Can you work these out from the model? Positions are in its coordinate system, mm. Face numbers are marked on the shaded views. A direction names the side the tool comes from. Round coordinates to 2 decimals unless told otherwise and drop trailing zeros. Write each loop counter-clockwise with the first axis right and the second up, starting at its lowest first coordinate (ties: lowest second). Pieces come first, ordered by that corner, then holes. Notation, with made-up numbers: M 0,25.5 L 47,25.5 A28 cw 47,60.5 Z; hole C 40.5,25.5 d2. An arc over 180 degrees is marked long. Answer as a JSON object with one key per item and string values. Group by question number.
1) Suppose I cut it at C-C, the plane z = 7. Write out the boundary of the cut face in (x, y), and give its area (3 significant figures).
2) I'm going to push flat-ended pins straight in: pin 1 Ø1 at (x, y) = (-10.5, -10) entering from +Z; pin 2 Ø2 at (y, z) = (18.5, 4) entering from -X; pin 3 Ø8 at (y, z) = (-21, 5) entering from -X; pin 4 Ø1.5 at (x, y) = (24, -21.5) entering from -Z. Where does each tip first touch, or does it pass through?
3) On a 3-axis mill with a long thin cutter (end or side, diameter ignored), from which of +Z, -Z, +X, -X, +Y, -Y can I reach the whole of each face in a straight line? I mean the marked faces 4, 5 and 6. Say none if no direction works.
4) Please list where these lines run through material, in increasing order: L1, parallel to Z at x = 15.5, y = 23; L2, parallel to Z at x = -6.5, y = -14.5; L3, parallel to Y at x = -7.5, z = -7.25. Write a range as [from, to].
5) Suppose I cut it at B-B, the plane x = 0. Write out the boundary of the cut face in (y, z).
6) Suppose I cut it at A-A, the plane y = 0. Write out the boundary of the cut face in (x, z), and give its area (3 significant figures).
7) If we mould it in two halves opening along X, with no side actions, what happens to the marked faces 1, 2 and 3? For each: +X half, -X half, draft (parallel to the pull), parting line (faces both ways), or undercut.
8) Suppose I cut it at D-D, the plane y = 20. Write out the boundary of the cut face in (x, z).
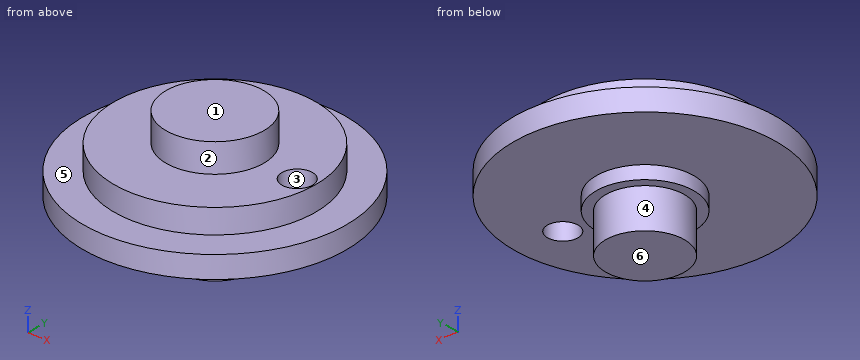
from build123d import *

# Parameters (mm, degrees)
F0_R          = 30
F1_DEPTH      = 5
F2_R          = 11.15
F3_DEPTH      = 12
F3_DEPTH_BACK = 8
F4_R          = 9
F5_DEPTH      = 9
F6_R          = 23
F7_DEPTH      = 5.5
F8_R          = 3.5
F9_DEPTH      = 12.5


with BuildPart() as f1:
    # F0 (on Top) → F1 (new body)
    with BuildSketch(Plane.XY):
        Circle(F0_R)
    extrude(amount=F1_DEPTH)

    # F2 (on face) → F3 (join, two sides)
    with BuildSketch(Plane.XY.offset(5)) as f3_sk:
        Circle(F2_R)
    extrude(amount=F3_DEPTH)
    extrude(f3_sk.sketch, amount=-F3_DEPTH_BACK)

    # F4 (on face) → F5 (join)
    with BuildSketch(Plane(origin=(0, 0, -3), x_dir=(1, 0, 0), z_dir=(0, 0, -1))):
        Circle(F4_R)
    extrude(amount=F5_DEPTH)

    # F6 (on face) → F7 (join)
    with BuildSketch(Plane.XY.offset(5)):
        Circle(F6_R)
    extrude(amount=F7_DEPTH)

    # F8 (on face) → F9 (cut, symmetric)
    with BuildSketch(Plane.XY.offset(5)):
        with Locations((19.200256, 0)):
            Circle(F8_R)
    extrude(amount=F9_DEPTH, both=True, mode=Mode.SUBTRACT)


solid = f1.part
Results:
{
 "1": {"outline": "C 0,0 d46; hole C 19.2,0 d7", "area": "1,620 mm^2"},
 "2": {"pin 1": "z = 10.5", "pin 2": "x = -24.37", "pin 3": "x = -24.72", "pin 4": "through"},
 "3": {"face 4": "-Z", "face 5": "+Z", "face 6": "-Z, +X, -X, +Y, -Y"},
 "4": {"L1": "[0, 5]", "L2": "[0, 10.5]", "L3": "[-4.97, 4.97]"},
 "5": {"outline": "M -30,0 L -11.15,0 L -11.15,-3 L -9,-3 L -9,-12 L 9,-12 L 9,-3 L 11.15,-3 L 11.15,0 L 30,0 L 30,5 L 23,5 L 23,10.5 L 11.15,10.5 L 11.15,17 L -11.15,17 L -11.15,10.5 L -23,10.5 L -23,5 L -30,5 Z"},
 "6": {"outline": "M -30,0 L -11.15,0 L -11.15,-3 L -9,-3 L -9,-12 L 9,-12 L 9,-3 L 11.15,-3 L 11.15,0 L 15.7,0 L 15.7,10.5 L 11.15,10.5 L 11.15,17 L -11.15,17 L -11.15,10.5 L -23,10.5 L -23,5 L -30,5 Z; M 22.7,0 L 30,0 L 30,5 L 23,5 L 23,10.5 L 22.7,10.5 Z", "area": "853 mm^2"},
 "7": {"face 1": "draft", "face 2": "parting line", "face 3": "undercut"},
 "8": {"outline": "M -22.36,0 L 22.36,0 L 22.36,5 L 11.36,5 L 11.36,10.5 L -11.36,10.5 L -11.36,5 L -22.36,5 Z"}
}
